Part model, mm, in its own coordinate system. Face numbers are marked on the shaded views. A direction names the side the tool comes from. Round coordinates to 2 decimals unless told otherwise and drop trailing zeros. Loops run counter-clockwise (first coordinate to the right, second up) from the corner with the lowest first, then second, coordinate; pieces in that order, holes last. Notation, with made-up numbers: (1.25, 41.5) -> (25.25, 41.5) arc R16 ccw to (25.25, 50.5) -> close; hole circle Ø10 at (-30.75, 62). An arc over 180 degrees is marked (long way). Use a Markdown table: item, result. Add a question column.
Item 1: Cut at A-A, the plane x = -7. List the corners of the cut face in (y, z), plus the area to 3 significant figures.
Item 2: Cut at B-B, the plane x = -16.5. List the corners of the cut face in (y, z).
Item 3: Cut at C-C, the plane z = -0.75. List the corners of the cut face in (x, y).
Item 4: Flat gauge pins, fed straight in: pin 1 (3.5 mm diameter, centred on y = -5, z = 4, fed in from +X); pin 2 (3.5 mm diameter, centred on x = 13, z = -0.75, fed in from -Y); pin 3 (4 mm diameter, centred on x = 0.5, y = 6.5, fed in from +Z). Where does each tip first touch, or does it go through?
Item 5: Probe line 1 (Z direction, x = -16.5, y = 7.65); line 2 (Z direction, x = 13, y = 0.6); line 3 (Y direction, x = -16, z = 5.5). List the from-to ranges inside material, lowest first. Write a range as [from, to].
Item 6: Cut at D-D, the plane z = -5. List the corners of the cut face in (x, y).
Item 7: Two-plate mould, pull along X, no slides. Class the marked faces 6, 7 and 8: pulls with the +X half, pulls with the -X half, needs draft (parallel to the pull), parting line crosses it, or undercut.
Item 8: Which spindle directions (+Z, -Z, +X, -X, +Y, -Y) get a long thin tool onto all of the face, cutting with end or side? Do the marked faces 1, 2, 3, 4 and 5. Say none if no direction does.
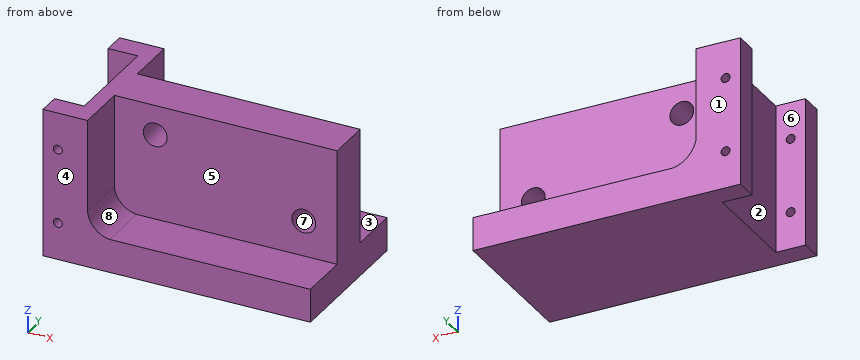
```python
from build123d import *

# Parameters (mm, degrees)
SKETCH1_W           = 35
SKETCH1_H           = 20
BOSS_EXTRUDE2_DEPTH = 10
CUT_EXTRUDE1_DEPTH  = 7
CUT_EXTRUDE2_DEPTH  = 7
SKETCH8_R           = 1.6
CUT_EXTRUDE3_DEPTH  = 7
SKETCH9_W           = 20
SKETCH9_H           = 14
CUT_EXTRUDE4_DEPTH  = 3
SKETCH10_R          = 0.6
CUT_EXTRUDE5_DEPTH  = 3
SKETCH11_R          = 0.6
CUT_EXTRUDE6_DEPTH  = 3
SKETCH12_W          = 20
SKETCH12_H          = 3
BOSS_EXTRUDE3_DEPTH = 1
SKETCH13_W          = 20
SKETCH13_H          = 3
BOSS_EXTRUDE4_DEPTH = 1


with BuildPart() as part:
    # Sketch1 → Boss-Extrude2 (new body, symmetric)
    with BuildSketch(Plane(origin=(0, 0, 0), x_dir=(1, 0, 0), z_dir=(0, 1, 0))):
        Rectangle(SKETCH1_W, SKETCH1_H)
    extrude(amount=BOSS_EXTRUDE2_DEPTH, both=True)

    # Sketch4 → Cut-Extrude1 (cut)
    with BuildSketch(Plane(origin=(0, 10, 0), x_dir=(1, 0, 0), z_dir=(0, 1, 0))):
        with BuildLine():
            Line((-12.5, -10), (-12.5, 2.5))
            ThreePointArc((-12.5, 2.5), (-11.447225408, 4.447225408), (-9.5, 5.5))
            Line((-9.5, 5.5), (17.5, 5.5))
            Line((17.5, 5.5), (17.5, -10))
            Line((17.5, -10), (-12.5, -10))
        make_face()
    extrude(amount=-CUT_EXTRUDE1_DEPTH, mode=Mode.SUBTRACT)

    # Sketch6 → Cut-Extrude2 (cut)
    with BuildSketch(Plane.XZ.offset(10)):
        with BuildLine():
            Line((-12.5, 10), (-12.5, -2.5))
            ThreePointArc((-12.5, -2.5), (-11.528297563, -4.528297563), (-9.5, -5.5))
            Line((-9.5, -5.5), (17.5, -5.5))
            Line((17.5, -5.5), (17.5, 10))
            Line((17.5, 10), (-12.5, 10))
        make_face()
    extrude(amount=-CUT_EXTRUDE2_DEPTH, mode=Mode.SUBTRACT)

    # Sketch8 → Cut-Extrude3 (cut)
    with BuildSketch(Plane(origin=(0, 3, 0), x_dir=(1, 0, 0), z_dir=(0, 1, 0))):
        with Locations((-7, -6)):
            Circle(SKETCH8_R)
        with Locations((13, 0.75)):
            Circle(SKETCH8_R)
    extrude(amount=-CUT_EXTRUDE3_DEPTH, mode=Mode.SUBTRACT)

    # Sketch9 → Cut-Extrude4 (cut)
    with BuildSketch(Plane.ZY.offset(17.5)):
        Rectangle(SKETCH9_W, SKETCH9_H)
    extrude(amount=-CUT_EXTRUDE4_DEPTH, mode=Mode.SUBTRACT)

    # Sketch10 → Cut-Extrude5 (cut)
    with BuildSketch(Plane(origin=(0, 10, 0), x_dir=(1, 0, 0), z_dir=(0, 1, 0))):
        with Locations((-16.5, 5)):
            Circle(SKETCH10_R)
        with Locations((-16.5, -5)):
            Circle(SKETCH10_R)
    extrude(amount=-CUT_EXTRUDE5_DEPTH, mode=Mode.SUBTRACT)

    # Sketch11 → Cut-Extrude6 (cut)
    with BuildSketch(Plane.XZ.offset(10)):
        with Locations((-16.5, 5)):
            Circle(SKETCH11_R)
        with Locations((-16.5, -5)):
            Circle(SKETCH11_R)
    extrude(amount=-CUT_EXTRUDE6_DEPTH, mode=Mode.SUBTRACT)

    # Sketch12 → Boss-Extrude3 (add)
    with BuildSketch(Plane.ZY.offset(17.5)):
        with Locations((0, 8.5)):
            Rectangle(SKETCH12_W, SKETCH12_H)
    extrude(amount=BOSS_EXTRUDE3_DEPTH)

    # Sketch13 → Boss-Extrude4 (add)
    with BuildSketch(Plane.ZY.offset(17.5)):
        with Locations((0, -8.5)):
            Rectangle(SKETCH13_W, SKETCH13_H)
    extrude(amount=BOSS_EXTRUDE4_DEPTH)


solid = part.part
```
A:
| question | item | result |
|---|---|---|
| 1 | outline | (-10, -10) -> (10, -10) -> (10, -5.5) -> (3, -5.5) -> (3, 4.4) -> (-3, 4.4) -> (-3, -5.5) -> (-10, -5.5) -> close; (-3, 7.6) -> (3, 7.6) -> (3, 10) -> (-3, 10) -> close |
| 1 | area | 164 mm^2 |
| 2 | outline | (-10, -10) -> (-7, -10) -> (-7, -5.6) -> (-10, -5.6) -> close; (-10, -4.4) -> (-7, -4.4) -> (-7, 4.4) -> (-10, 4.4) -> close; (-10, 5.6) -> (-7, 5.6) -> (-7, 10) -> (-10, 10) -> close; (7, -10) -> (10, -10) -> (10, -5.6) -> (7, -5.6) -> close; (7, -4.4) -> (10, -4.4) -> (10, 4.4) -> (7, 4.4) -> close; (7, 5.6) -> (10, 5.6) -> (10, 10) -> (7, 10) -> close |
| 3 | outline | (-18.5, -10) -> (-12.5, -10) -> (-12.5, -3) -> (11.4, -3) -> (11.4, 3) -> (-12.5, 3) -> (-12.5, 10) -> (-18.5, 10) -> (-18.5, 7) -> (-14.5, 7) -> (-14.5, -7) -> (-18.5, -7) -> close; (14.6, -3) -> (17.5, -3) -> (17.5, 3) -> (14.6, 3) -> close |
| 4 | pin 1 | stops at x = -12.5 |
| 4 | pin 2 | stops at y = -3 |
| 4 | pin 3 | stops at z = -5.5 |
| 5 | line 1 | z = [-10, -5.6], [-4.4, 4.4], [5.6, 10] |
| 5 | line 2 | z = [-10, -2.35], [0.85, 10] |
| 5 | line 3 | y = [-10, -7], [7, 10] |
| 6 | outline | (-18.5, -10) -> (-17.1, -10) -> (-17.1, -7) -> (-18.5, -7) -> close; (-18.5, 7) -> (-17.1, 7) -> (-17.1, 10) -> (-18.5, 10) -> close; (-15.9, -10) -> (-10.94, -10) -> (-10.94, -3) -> (17.5, -3) -> (17.5, 3) -> (-10.75, 3) -> (-10.75, 10) -> (-15.9, 10) -> (-15.9, 7) -> (-14.5, 7) -> (-14.5, -7) -> (-15.9, -7) -> close |
| 7 | face 6 | needs draft |
| 7 | face 7 | undercut |
| 7 | face 8 | pulls with the +X half |
| 8 | face 1 | +Z, -Z, +X, -X, +Y |
| 8 | face 2 | +Z, -Z, -X |
| 8 | face 3 | +Z, +X, +Y |
| 8 | face 4 | +Z, -Z, +X, -X, -Y |
| 8 | face 5 | +Z, +X, -Y |
